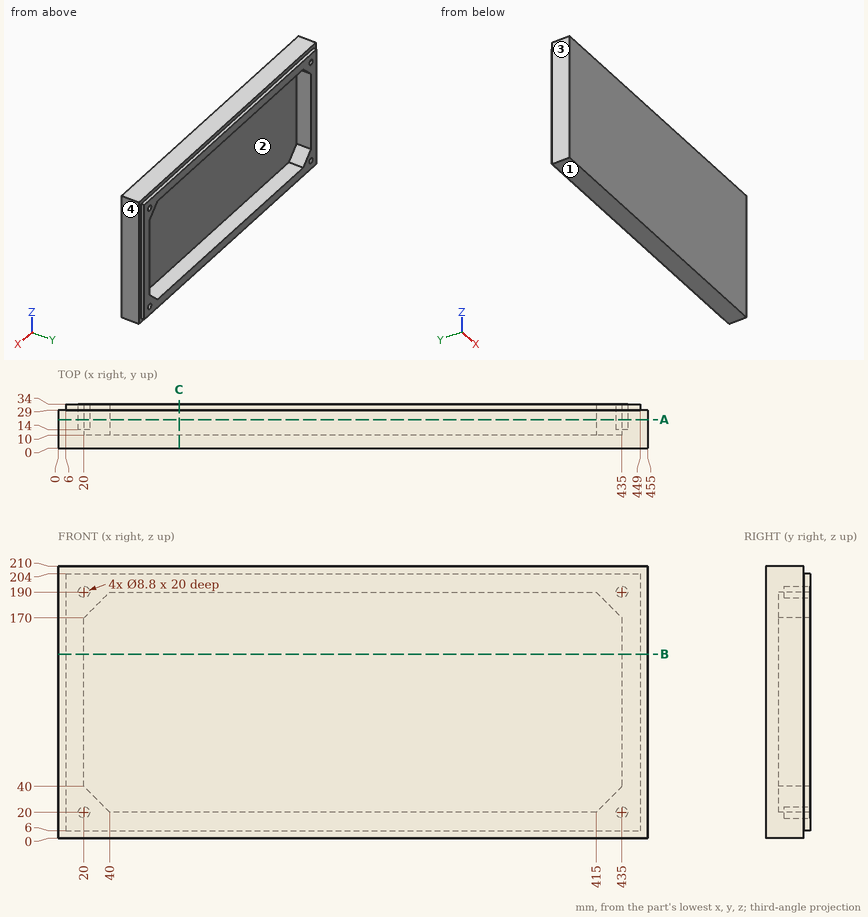
The figure shows three views and two pictorial views of one solid part (mm, origin at its lowest corner). Answer the questions. Round coordinates to 2 decimals unless told otherwise and drop trailing zeros. Loops run counter-clockwise (first coordinate to the right, second up) from the corner with the lowest first, then second, coordinate; pieces in that order, holes last. Notation, with made-up numbers: M 78.5,26 L 93.5,26 A13 cw 93.5,51 Z; hole C 21,74 d9. An arc over 180 degrees is marked long. Write each question's results on one line, items separated by ' | '. Start each with the question number.
1) Straight lines are drawn through the part: probe 1 along Z at (x, y) = (70, 24); probe 2 along X at (y, z) = (24, 87); probe 3 along X at (y, z) = (31.5, 70). For each, find the intervals that lie inside material, in ascending order.
2) Each of these flat-tipped pins is pushed along its axis until it touches: pin 1 (5.5 mm diameter, centred on x = 127, y = 32.5, fed in from -Z); pin 2 (8 mm diameter, centred on x = 194, z = 84, fed in from +Y); pin 3 (2.5 mm diameter, centred on y = 31.5, z = 144, fed in from +X). Where does it stop, or does it pass through?
3) Determine the mould class of the marked faces 1, 2, 3 and 4 for opening direction X: pulls with the +X half, pulls with the -X half, needs draft (parallel to the pull), parting line crosses it, or undercut.
4) Find section C-C on x = 93.5. Write down the section's boundary in (y, z).
5) Find section A-A on y = 22. Write down the section's boundary in (x, z).
6) Find section B-B on z = 142. Write down the section's boundary in (x, y), plus the area to 3 significant figures.
Final values:
1) probe 1: 0 to 20, 190 to 210 | probe 2: 0 to 20, 435 to 455 | probe 3: 6 to 20, 435 to 449
2) pin 1: z = 6 | pin 2: y = 10 | pin 3: x = 449
3) face 1: needs draft | face 2: undercut | face 3: pulls with the -X half | face 4: pulls with the +X half
4) outline: M 0,0 L 29,0 L 29,6 L 34,6 L 34,20 L 10,20 L 10,190 L 34,190 L 34,204 L 29,204 L 29,210 L 0,210 Z
5) outline: M 0,0 L 455,0 L 455,210 L 0,210 Z; hole C 20,20 d8.8; hole C 20,190 d8.8; hole M 20,40 L 40,20 L 415,20 L 435,40 L 435,170 L 415,190 L 40,190 L 20,170 Z; hole C 435,20 d8.8; hole C 435,190 d8.8
6) outline: M 0,0 L 455,0 L 455,29 L 449,29 L 449,34 L 435,34 L 435,10 L 20,10 L 20,34 L 6,34 L 6,29 L 0,29 Z | area: 5,450 mm²
